Verification items for this drawing (mm, ordinates from the low corner). Give positions to 0.01 mm unless a question says otherwise; leave off trailing zeros. Loops run counter-clockwise (first coordinate to the right, second up) from the corner with the lowest first, then second, coordinate; pieces in that order, holes last. Notation, with made-up numbers: (69, -19) -> (102, -19) arc R24 cw to (102, 0) -> close; hole circle Ø4 at (76, 9.5). An arc over 180 degrees is marked (long way). Answer as a JSON object with one key per item and string values.
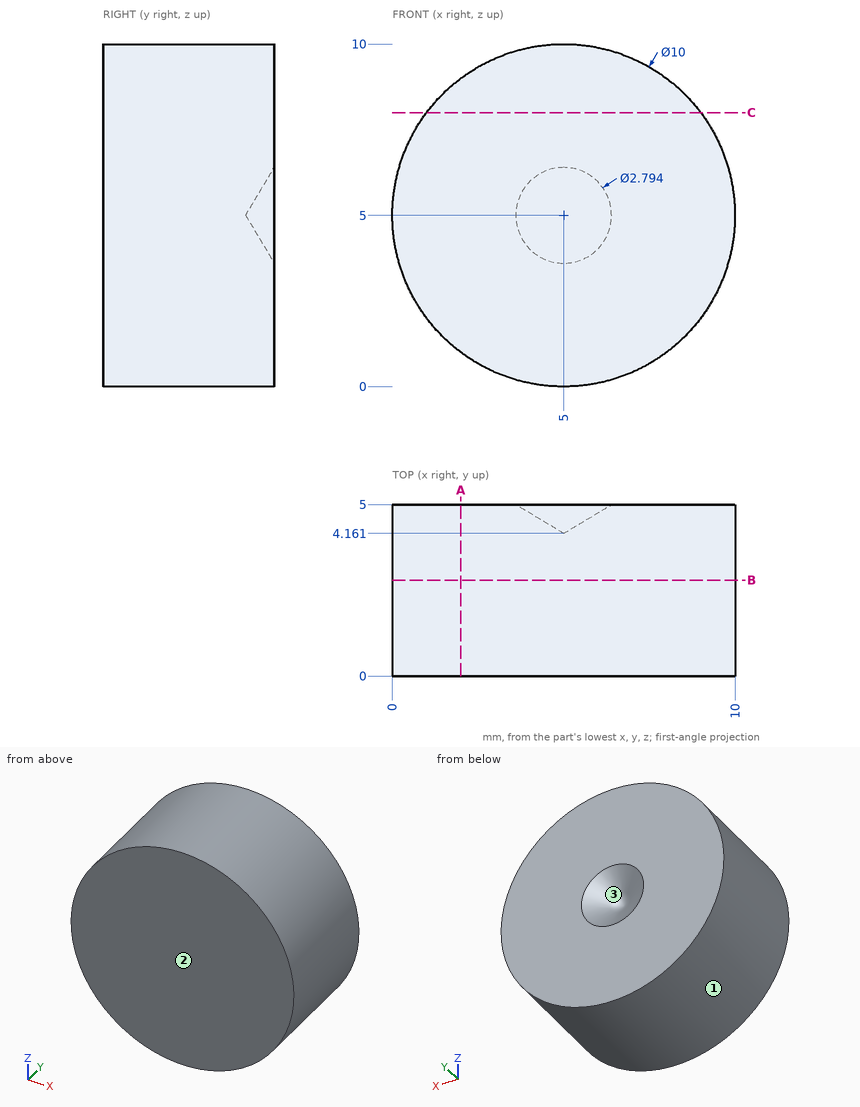
1) Section check A-A on x = 2. Record the cut outline in (y, z).
Geometry check:
{"outline": "(0, 1) -> (5, 1) -> (5, 9) -> (0, 9) -> close"}
2) Section check C-C on z = 8. Record the cut outline in (x, y), plus the area to 3 significant figures.
Geometry check:
{"outline": "(1, 0) -> (9, 0) -> (9, 5) -> (1, 5) -> close", "area": "40.0 mm2"}
3) Section check B-B on y = 2.8. Record the cut outline in (x, z).
Geometry check:
{"outline": "circle Ø10 at (5, 5)"}
4) Material ranges on line 1 along Z through (x, y) = (1, 2.35); line 2 along X through (y, z) = (0.85, 3.5); line 3 along X through (y, z) = (3.95, 9.5), recorded low to high. Write a range as from..to.
Geometry check:
{"line 1": "z = 2..8", "line 2": "x = 0.23..9.77", "line 3": "x = 2.82..7.18"}
5) Draft check along X on the marked faces 1, 2 and 3. Enter one of: pulls with the +X half, pulls with the -X half, needs draft (parallel to the pull), parting line crosses it, or undercut.
Geometry check:
{"face 1": "parting line crosses it", "face 2": "needs draft", "face 3": "undercut"}
